from build123d import *

# Parameters (mm, degrees)
F2_R     = 8
F3_DEPTH = 25


with BuildPart() as f1:
    # F0 (on Front) → F1 (revolve)
    with BuildSketch(Plane.XZ):
        Polygon((24.92856, 7.9248), (24.92856, 12.542502), (-8.72644, 12.542502), (-13.80644, 17.102293), (-13.80644, 20.379981), (-23.96644, 20.379981), (-23.96644, 2.599981), (-31.292418, 2.599981), (-31.292418, -5.020019), (4.60856, -5.020019), (4.60856, 5.08), (30.00856, 5.08), (30.00856, 7.9248), align=None)
    revolve(axis=Axis((-13.341929, 0, -5.020019), (1, 0, 0)))

    # F2 (on face) → F3 (cut)
    with BuildSketch(Plane(origin=(-23.96644, 0, 0), x_dir=(0, -1, 0), z_dir=(-1, 0, 0))):
        with BuildLine():
            ThreePointArc((8, 24.70155), (-5.656854, 30.358404), (0, 16.70155))
            ThreePointArc((0, 16.70155), (5.656854, 19.044696), (8, 24.70155))
        make_face()
        with BuildLine():
            ThreePointArc((8, -34.741588), (5.656854, -29.084734), (0, -26.741588))
            ThreePointArc((0, -26.741588), (-5.656854, -40.398442), (8, -34.741588))
        make_face()
        with Locations((-29.721569, -5.020019)):
            Circle(F2_R)
        with BuildLine():
            ThreePointArc((37.721569, -5.020019), (29.721569, 2.979981), (21.721569, -5.020019))
            ThreePointArc((21.721569, -5.020019), (29.721569, -13.020019), (37.721569, -5.020019))
        make_face()
        with BuildLine():
            ThreePointArc((-13.016323, 15.996304), (-28.407359, 19.057771), (-15.359469, 10.33945))
            ThreePointArc((-15.359469, 10.33945), (-13.625287, 12.934836), (-13.016323, 15.996304))
        make_face()
        with BuildLine():
            ThreePointArc((29.016323, 15.996304), (17.954856, 23.38734), (15.359469, 10.33945))
            ThreePointArc((15.359469, 10.33945), (24.07779, 8.605268), (29.016323, 15.996304))
        make_face()
        with BuildLine():
            ThreePointArc((29.016323, -26.036342), (24.07779, -18.645306), (15.359469, -20.379488))
            ThreePointArc((15.359469, -20.379488), (17.954856, -33.427378), (29.016323, -26.036342))
        make_face()
        with BuildLine():
            ThreePointArc((-13.379907, -25.666356), (-13.962437, -22.669503), (-15.625189, -20.109089))
            ThreePointArc((-15.625189, -20.109089), (-28.797378, -28.663208), (-13.379907, -25.666356))
        make_face()
    extrude(amount=-F3_DEPTH, mode=Mode.SUBTRACT)


solid = f1.part
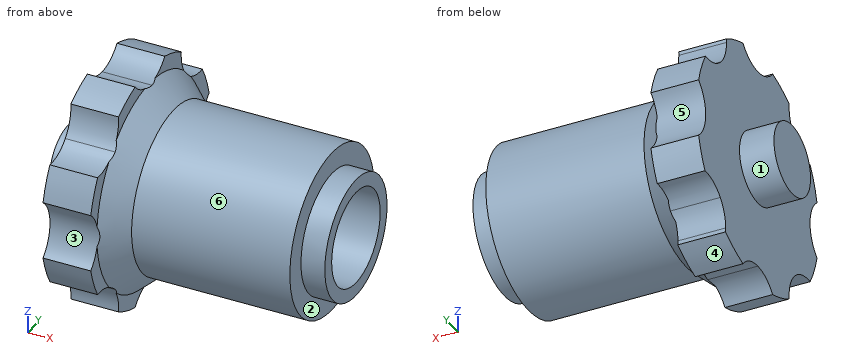
The model under review builds one solid part; all positions refer to its coordinate system, in mm. Face numbers are marked on the shaded views. A direction names the side the tool comes from. Coordinates: 2 decimals unless noted, no trailing zeros. Loops run counter-clockwise (first coordinate to the right, second up) from the corner with the lowest first, then second, coordinate; pieces in that order, holes last. Notation, with made-up numbers: (51, 49) -> (85, 49) arc R21 cw to (85, 53) -> close; hole circle Ø7 at (86.25, 65.25). An arc over 180 degrees is marked (long way). Use a Markdown table: item, result. Add a question column.
1. To check wall thickness, follow line 1 (Z direction, x = 10, y = 0); line 2 (X direction, y = -2, z = -6); line 3 (X direction, y = -1.5, z = -19.5). State the ranges of each line that lie inside material, in increasing order.
2. Add section B-B on x = -18. Write out the cut boundary in (y, z).
3. Draft analysis for pull direction Z (two halves, no side actions). For the marked faces 4, 5 and 6, state which applies: pulls with the +Z half, pulls with the -Z half, needs draft (parallel to the pull), parting line crosses it, or undercut.
4. Clearance check with flat-ended pins moving along their axes: pin 1 Ø8 at (x, z) = (-10, -21.5) entering from +Y; pin 2 Ø6 at (y, z) = (-20, 4) entering from +X; pin 3 Ø2 at (x, z) = (17, -10.5) entering from +Y. State where each tip first meets the part, or that it passes through.
5. Machinability: for the marked faces 1, 2 and 3, which of the approach directions +Z, -Z, +X, -X, +Y, -Y give a long, thin tool a straight path to every point of the face, cutting with its end or side? Answer none if there is none.
6. Add section C-C on x = 2.5. Write out the cut boundary in (y, z), plus the area to 3 significant figures.
7. Add section A-A on x = 21.5. Write out the cut boundary in (y, z), plus the area to 3 significant figures.
Returned:
| question | item | result |
|---|---|---|
| 1 | line 1 | z = -22.58 to -15.12, 5.08 to 12.54 |
| 1 | line 2 | x = -31.29 to 4.61 |
| 1 | line 3 | x = -23.97 to 24.93 |
| 2 | outline | (-24.64, -11.2) arc R25.4 ccw to (-21.79, -18.07) arc R8 cw to (-13.05, -26.81) arc R25.4 ccw to (-6.18, -29.66) arc R8 cw to (6.18, -29.66) arc R25.4 ccw to (13.43, -26.58) arc R8 cw to (13.38, -25.67) arc R8 cw to (15.63, -20.11) arc R8 cw to (22.01, -17.69) arc R25.4 ccw to (24.64, -11.2) arc R8 cw to (24.64, 1.16) arc R25.4 ccw to (21.79, 8.03) arc R8 cw to (15.36, 10.34) arc R8 cw to (13.02, 16) arc R8 cw to (13.05, 16.77) arc R25.4 ccw to (6.18, 19.62) arc R8 cw to (-6.18, 19.62) arc R25.4 ccw to (-13.05, 16.77) arc R8 cw to (-21.79, 8.03) arc R25.4 ccw to (-24.64, 1.16) arc R8 cw to start |
| 3 | face 4 | pulls with the -Z half |
| 3 | face 5 | undercut |
| 3 | face 6 | parting line crosses it |
| 4 | pin 1 | stops at y = 16.35 |
| 4 | pin 2 | stops at x = -10.26 |
| 4 | pin 3 | stops at y = 16.98 |
| 5 | face 1 | -X |
| 5 | face 2 | +X |
| 5 | face 3 | +X, -X, -Y |
| 6 | outline | circle Ø35.13 at (0, -5.02) |
| 6 | area | 969 mm² |
| 7 | outline | circle Ø35.13 at (0, -5.02); hole circle Ø20.2 at (0, -5.02) |
| 7 | area | 649 mm² |
